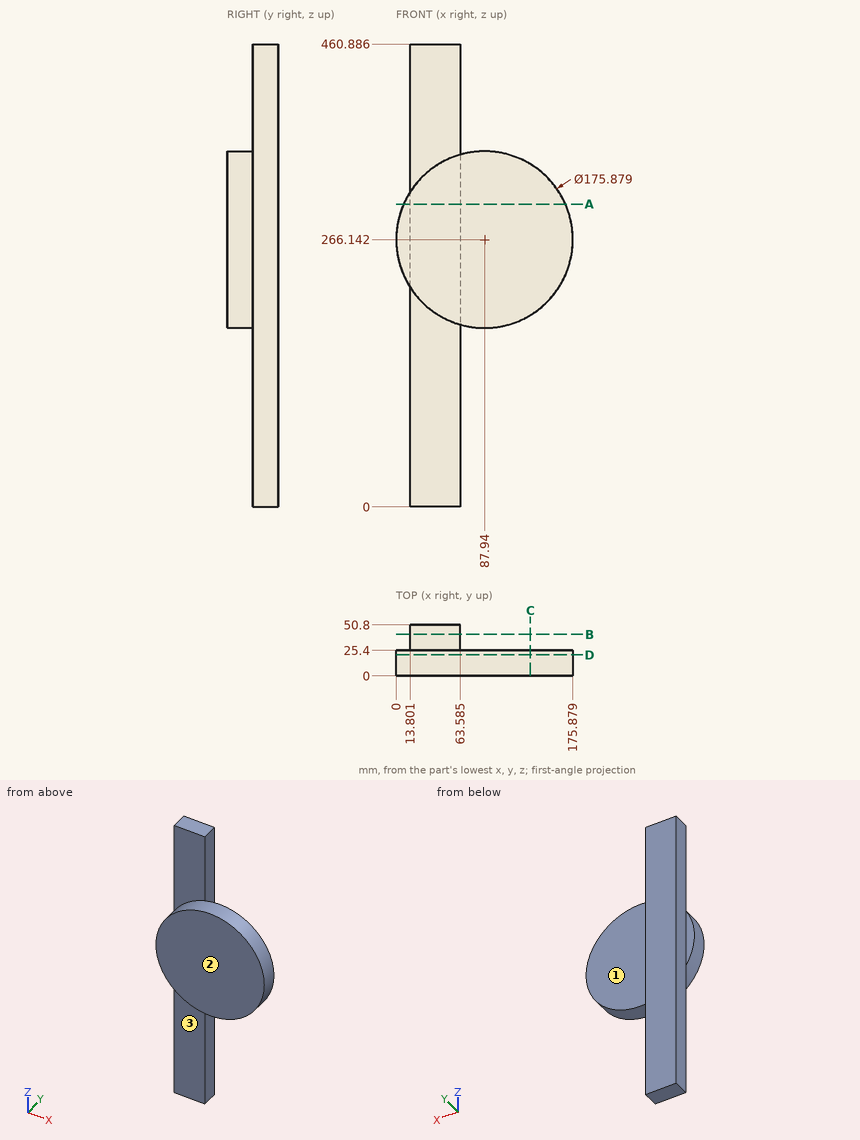
For this review, use the dimensioned drawing (mm, ordinates from the lowest corner) and the shaded views. A direction names the side the tool comes from. Give positions to 0.01 mm unless a question says otherwise; leave off trailing zeros. Loops run counter-clockwise (first coordinate to the right, second up) from the corner with the lowest first, then second, coordinate; pieces in that order, holes last.
Item 1: For line 1 along Y through (x, z) = (44, 358.5); line 2 along X through (y, z) = (30, 123) (1 decimal); line 3 along Y through (x, z) = (117, 346.5), list the stretches that pass through material, from the lowest coordinate up.
Item 2: Take a section at D-D, the plane y = 21. State the section outline as (x, z) points, and give its area (3 significant figures).
Item 3: Take a section at A-A, the plane z = 301.5. State the section outline as (x, y) points (1 decimal).
Item 4: Take a section at C-C, the plane x = 133.5. State the section outline as (y, z) points (1 decimal), and give its area (3 significant figures).
Item 5: Take a section at B-B, the plane y = 41.5. State the section outline as (x, z) points (1 decimal).
Item 6: Tool access review of the marked faces 1, 2 and 3: name each direction out of +Z, -Z, +X, -X, +Y, -Y from which nothing blocks a thin tool from reaching the whole face with its end or side.
Item 7: Insertion check: pin 1 (20.5 mm diameter, centred on y = 33, z = 132.5, fed in from -X); pin 2 (7.5 mm diameter, centred on y = 33, z = 331, fed in from +X) (1 decimal); pin 3 (12 mm diameter, centred on x = 119.5, z = 299.5, fed in from +Y). Each pin has a flat end and moves straight along its axis. Give the tip position at first contact, or say it passes through.
Calculated:
1. line 1: y = 25.4 to 50.8
1. line 2: x = 13.8 to 63.6
1. line 3: y = 0 to 25.4
2. outline: circle Ø175.88 at (87.94, 266.14)
2. area: 24,300 mm2
3. outline: (7.4, 0) - (168.5, 0) - (168.5, 25.4) - (63.6, 25.4) - (63.6, 50.8) - (13.8, 50.8) - (13.8, 25.4) - (7.4, 25.4) - close
4. outline: (0, 190.9) - (25.4, 190.9) - (25.4, 341.4) - (0, 341.4) - close
4. area: 3,820 mm2
5. outline: (13.8, 0) - (63.6, 0) - (63.6, 460.9) - (13.8, 460.9) - close
6. face 1: +Z, -Z, +X, +Y
6. face 2: +Z, -Z, +X, -X, -Y
6. face 3: -Z, -X, -Y
7. pin 1: stops at x = 13.8
7. pin 2: stops at x = 63.6
7. pin 3: stops at y = 25.4
